Solid Edge part; units mm, degrees
sketch "Sketch1" plane through (0, 0, 0) normal (0, 0, 1) x (1, 0, 0)
  line L0 (-6.5, -8) -> (6.5, -8)
  line L1 (6.5, -8) -> (6.5, 2)
  line L2 (-6.5, 2) -> (6.5, 2)
  line L3 (-6.5, -8) -> (-6.5, 2)
  dimension "D1" = 6.5
  dimension "D2" = 6.5
  dimension "D3" = 6.5
extrude "Ajout_matière_1" add sketch "Sketch1" along normal mid plane 100
hole "Hole1" at (0, -8, -19) direction (0, 1, 0) diameter 4.459 end up to next
hole "Hole2" at (0, -8, 23) direction (0, 1, 0) diameter 4.459 end up to next
hole "Hole3" at (0, -8, 2) direction (0, 1, 0) diameter 4.459 end up to next
hole "Hole4" at (0, -8, 44) direction (0, 1, 0) diameter 4.459 end up to next
sketch "Sketch2" plane through (0, 2, -50) normal (0, 0, -1) x (0, 1, 0)
  line L0 (-10, -6.5) -> (-2, -6.5)
  line L1 (-2, -6.5) -> (-2, -7.5)
  line L2 (-2, -7.5) -> (10, -7.5)
  line L3 (10, -7.5) -> (10, 7.5)
  line L4 (10, 7.5) -> (-2, 7.5)
  line L5 (-2, 7.5) -> (-2, 6.5)
  line L6 (-2, 6.5) -> (-10, 6.5)
  line L7 (-10, 6.5) -> (-10, -6.5)
extrude "Ajout_matière_3" add sketch "Sketch2" along normal mid plane 2.5
mirror "Mirror1" about plane through (0, 0, 0) normal (0, 0, 1) of "Ajout_matière_3"
hole "Perçage_2" at (0, 8, 51.25) direction (0, 0, -1) diameter 5 end through all
chamfer "Chamfer1" distance 1 angle 45 8 edges at (-7.5, 12, 50) (-7.5, 12, -50) (-6.5, 0, 50) (-6.5, 0, -50) (6.5, 0, 50) (6.5, 0, -50) (7.5, 12, 50) (7.5, 12, -50)
hole "Perçage_6" at (0, -8, -12.5) direction (0, 1, 0) diameter 3.242 end up to next
hole "Hole5" at (0, -8, 12.5) direction (0, 1, 0) diameter 3.242 end up to next
hole "Hole6" at (0, -8, -37.5) direction (0, 1, 0) diameter 3.242 end up to next
hole "Hole7" at (0, -8, 37.5) direction (0, 1, 0) diameter 3.242 end up to next
properties material "Aluminium AU4G, 2024_T4"
Build history of the part. All positions in model axes, mm. A direction names the side the tool comes from. Round coordinates to 2 decimals unless told otherwise and drop trailing zeros. Loops run counter-clockwise (first coordinate to the right, second up) from the corner with the lowest first, then second, coordinate; pieces in that order, holes last. Notation, with made-up numbers: (19, 49) -> (75, 49) arc R17 cw to (75, 55) -> close; hole circle Ø1 at (34.25, -9.75). An arc over 180 degrees is marked (long way). Answer in a Markdown table with one row per item.
Item 1: Saw through at A-A (y = 3.25). Write the cut outline in (x, z), and give its area (3 significant figures).
Answers below:
| item | result |
|---|---|
| outline | (-7.5, -51.25) -> (7.5, -51.25) -> (7.5, -48.75) -> (-7.5, -48.75) -> close; (-7.5, 48.75) -> (7.5, 48.75) -> (7.5, 51.25) -> (-7.5, 51.25) -> close |
| area | 75.0 mm² |
Item 2: Drill centre lines: L1, parallel to Z at x = -5, y = 6.25; L2, parallel to X at y = -4.5, z = -12.5; L3, parallel to X at y = -1, z = 2. Where is each one in solid material? Low to high. Write a range as [from, to].
Answers below:
| item | result |
|---|---|
| L1 | z = [-51.25, -48.75], [48.75, 51.25] |
| L2 | x = [-6.5, -1.62], [1.62, 6.5] |
| L3 | x = [-6.5, -2.23], [2.23, 6.5] |
Item 3: Which spindle directions (+Z, -Z, +X, -X, +Y, -Y) get a long thin tool onto all of the face, cutting with end or side? Do faces 1 (the flat face through (0, 2, -1)), 2 (the flat face through (0, 12, -50)). Say none if no direction does.
Answers below:
| item | result |
|---|---|
| face 1 | +X, -X, +Y |
| face 2 | +Z, -Z, +X, -X, +Y |
Item 4: Saw through at D-D (y = 8). Write the cut outline in (x, z), and give its area (3 significant figures).
Answers below:
| item | result |
|---|---|
| outline | (-7.5, -51.25) -> (-2.5, -51.25) -> (-2.5, -48.75) -> (-7.5, -48.75) -> close; (-7.5, 48.75) -> (-2.5, 48.75) -> (-2.5, 51.25) -> (-7.5, 51.25) -> close; (2.5, -51.25) -> (7.5, -51.25) -> (7.5, -48.75) -> (2.5, -48.75) -> close; (2.5, 48.75) -> (7.5, 48.75) -> (7.5, 51.25) -> (2.5, 51.25) -> close |
| area | 50.0 mm² |
Item 5: Saw through at B-B (z = 23). Write the cut outline in (x, y).
Answers below:
| item | result |
|---|---|
| outline | (-6.5, -8) -> (-2.23, -8) -> (-2.23, 2) -> (-6.5, 2) -> close; (2.23, -8) -> (6.5, -8) -> (6.5, 2) -> (2.23, 2) -> close |
Item 6: Pin check, flat tips, straight feed: pin 1 (7 mm diameter, centred on x = 0, z = 2, fed in from -Y); pin 2 (1.5 mm diameter, centred on y = -2, z = 34.5, fed in from -X); pin 3 (6 mm diameter, centred on x = 0, z = -19, fed in from +Y); pin 4 (1.9 mm diameter, centred on x = 0, z = 12.5, fed in from -Y). Stop position of each tip, or through.
Answers below:
| item | result |
|---|---|
| pin 1 | stops at y = -8 |
| pin 2 | stops at x = -6.5 |
| pin 3 | stops at y = 2 |
| pin 4 | passes through |
Item 7: Mould opens along Z. For faces 3 (the flat face through (0, 2, 51.25)), 4 (the cylindrical face through (0.098, -3.07, -16.773)), 5 (the flat face through (0, 2, -51.25)), 6 (the flat face through (7.5, 6, -50)) say: +Z half, -Z half, draft (parallel to the pull), parting line (faces both ways), or undercut.
Answers below:
| item | result |
|---|---|
| face 3 | +Z half |
| face 4 | undercut |
| face 5 | -Z half |
| face 6 | draft |
Item 8: Saw through at C-C (y = -2.75). State how many separate pieces and enclosed holes the cut face has, and give its area (3 significant figures).
Answers below:
| item | result |
|---|---|
| separate pieces | 1 |
| enclosed holes | 8 |
| area | 1,240 mm² |
